from build123d import *

# Parameters (mm, degrees)
SKETCH1_R           = 1.4224
BOSS_EXTRUDE1_DEPTH = 3.048


with BuildPart() as part:
    # Sketch1 → Boss-Extrude1 (new body)
    with BuildSketch(Plane(origin=(0, 0, 0), x_dir=(1, 0, 0), z_dir=(0, 1, 0))):
        with BuildLine():
            ThreePointArc((76.670362462, 20.543761705), (56.126600757, 56.126600757), (20.543761705, 76.670362462))
            Line((20.543761705, 76.670362462), (17.256759832, 64.403104468))
            ThreePointArc((17.256759832, 64.403104468), (47.146344636, 47.146344636), (64.403104468, 17.256759832))
            Line((64.403104468, 17.256759832), (76.670362462, 20.543761705))
        make_face()
        with Locations((67.466302862, 27.945457648)):
            Circle(SKETCH1_R, mode=Mode.SUBTRACT)
        with Locations((27.945457648, 67.466302862)):
            Circle(SKETCH1_R, mode=Mode.SUBTRACT)
        with Locations((51.636472696, 51.636472696)):
            Circle(SKETCH1_R, mode=Mode.SUBTRACT)
    extrude(amount=BOSS_EXTRUDE1_DEPTH)


solid = part.part
The listing builds one solid part. Answer for the finished solid, in the listing's coordinates (mm). Coordinates: 2 decimals unless noted, no trailing zeros. Loops run counter-clockwise (first coordinate to the right, second up) from the corner with the lowest first, then second, coordinate; pieces in that order, holes last. Notation, with made-up numbers: (72.25, -7) -> (82.25, -7) arc R35 cw to (82.25, 28) -> close; hole circle Ø11 at (-7.5, 75.5). An arc over 180 degrees is marked (long way). Write item = value, one per line. Start each with the question number.
1) A cutting plane is placed at B-B (y = 1.1). Give the vertices of the cut face in (x, z) (3 decimals), then the cut area to 3 significant figures.
2) Given pin 1 Ø1 at (x, y) = (44.5, 0.5) entering from -Z; pin 2 Ø3.5 at (x, z) = (27.95, -67.47) entering from -Y; pin 3 Ø1.5 at (x, y) = (32.5, 0.5) entering from -Z, each flat-ended and moving along its own axis, determine where each tip first touches the part or whether it passes through.
3) A cutting plane is placed at C-C (z = -37.5). Give the vertices of the cut face in (x, y), then the cut area to 3 significant figures.
4) The mould has two halves that part along X. Classify faces 1 (the face through (49, 0, -47)), 2 (the face through (46.8, 1.5, -47.49)), 3 (the face through (68.823, 1.503, -28.373)), 4 (the face through (51.328, 1.503, -50.248)): released by +X, released by -X, zero draft, split by the parting line, or undercut.
5) A cutting plane is placed at D-D (x = 28). Give the vertices of the cut face in (y, z), then the cut area to 3 significant figures.
6) A cutting plane is placed at A-A (x = 52). Give the vertices of the cut face in (y, z).
7) Straight lines are drawn through the part: line 1 (Z direction, x = 29, y = 1.35); line 2 (Z direction, x = 27.5, y = 1.05); line 3 (X direction, y = 0.95, z = -66.5). For each, find the intervals that lie inside material, in ascending order. Write a range as from..to.
Responses:
q1.outline = (17.257, -64.403) -> (20.544, -76.67) arc R79.375 ccw to (76.67, -20.544) -> (64.403, -17.257) arc R66.675 cw to start; hole circle Ø2.845 at (27.945, -67.466); hole circle Ø2.845 at (51.636, -51.636); hole circle Ø2.845 at (67.466, -27.945)
q1.area = 952 mm²
q2.pin_1 = -66.06
q2.pin_2 = 0
q2.pin_3 = -72.75
q3.outline = (55.13, 0) -> (69.96, 0) -> (69.96, 3.05) -> (55.13, 3.05) -> close
q3.area = 45.2 mm²
q4.face_1 = zero draft
q4.face_2 = released by -X
q4.face_3 = undercut
q4.face_4 = undercut
q5.outline = (0, -74.27) -> (3.05, -74.27) -> (3.05, -68.89) -> (0, -68.89) -> close; (0, -66.04) -> (3.05, -66.04) -> (3.05, -60.51) -> (0, -60.51) -> close
q5.area = 33.3 mm²
q6.outline = (0, -59.97) -> (3.05, -59.97) -> (3.05, -53.01) -> (0, -53.01) -> close; (0, -50.26) -> (3.05, -50.26) -> (3.05, -41.73) -> (0, -41.73) -> close
q7.line_1 = -73.89..-68.42, -66.51..-60.04
q7.line_2 = -74.46..-68.82, -66.12..-60.74
q7.line_3 = 17.82..26.9, 28.99..43.34
